```python
from build123d import *

# Parameters (mm, degrees)
SKETCH_1_W          = 86
SKETCH_1_H          = 44.4
EXTRUDE_1_DEPTH     = 19.6
EXTRUDE_2_DEPTH     = 5
SKETCH_3_W          = 83.2
SKETCH_3_H          = 20.402884615
SKETCH_3_H_2        = 20.397115385
CUT_EXTRUDE_1_DEPTH = 18.4
FILLET_1_R          = 3


with BuildPart() as part:
    # Эскиз1 → Бобышка-Вытянуть1 (new body)
    with BuildSketch(Plane.XY):
        Rectangle(SKETCH_1_W, SKETCH_1_H)
    extrude(amount=EXTRUDE_1_DEPTH)

    # Эскиз2 → Бобышка-Вытянуть2 (add)
    with BuildSketch(Plane.XY):
        with BuildLine():
            Line((43, 17.2), (43, 13.108775687))
            ThreePointArc((43, 13.108775687), (53.273546839, 0), (43, -13.108775687))
            Line((43, -13.108775687), (43, -17.2))
            ThreePointArc((43, -17.2), (57.273546839, 0), (43, 17.2))
        make_face()
    extrude(amount=EXTRUDE_2_DEPTH)

    # Эскиз3 → Вырез-Вытянуть1 (cut)
    with BuildSketch(Plane.XY.offset(19.6)):
        with Locations((0.2, 10.798557692)):
            Rectangle(SKETCH_3_W, SKETCH_3_H)
        with Locations((0.2, -10.801442308)):
            Rectangle(SKETCH_3_W, SKETCH_3_H_2)
    extrude(amount=-CUT_EXTRUDE_1_DEPTH, mode=Mode.SUBTRACT)

    # Скругление1
    fillet_1_edges = [part.edges().sort_by_distance(p)[0] for p in [
        (-41.4, 21, 10.4),
        (-41.4, -21, 10.4),
        (-43, -22.2, 9.8),
        (-43, 22.2, 9.8),
    ]]
    fillet(fillet_1_edges, radius=FILLET_1_R)


solid = part.part
```
Read the model definition and answer for the solid it produces. Units are mm, in the model's axes. A direction names the side the tool comes from. Coordinates: 2 decimals unless noted, no trailing zeros. Write each loop counter-clockwise with the first axis right and the second up, starting at its lowest first coordinate (ties: lowest second). Pieces come first, ordered by that corner, then holes. Notation, with made-up numbers: (-17.75, 40) -> (30.25, 40) arc R23 cw to (30.25, 60) -> close; hole circle Ø4 at (8.5, 19). An arc over 180 degrees is marked (long way). Write item = value, one per line.
(1) Section D-D on y = 1.5 is taken. Write down the section's boundary in (x, z).
From the geometry:
outline = (-43, 0) -> (43, 0) -> (43, 19.6) -> (41.8, 19.6) -> (41.8, 1.2) -> (-41.4, 1.2) -> (-41.4, 19.6) -> (-43, 19.6) -> close; (53.19, 0) -> (57.21, 0) -> (57.21, 5) -> (53.19, 5) -> close
(2) For a pull along X with two mould halves and no side action, classify faces 1 (the face through (1, 21, 11)), 2 (the face through (57.27, -0.34, 2.46)), 3 (the face through (-42.14, -21.3, 9.94)), 4 (the face through (1, 22.2, 10)) as +X half, -X half, draft (parallel to the pull), parting line (faces both ways), or undercut.
From the geometry:
face_1 = undercut
face_2 = +X half
face_3 = -X half
face_4 = draft
(3) Straight lines are drawn through the part: L1, parallel to Y at x = 16, z = 10.5; L2, parallel to X at y = 18, z = 12.5; L3, parallel to X at y = 3, z = 2. For each, find the intervals that lie inside material, in ascending order. Write a range as from..to.
From the geometry:
L1 = -22.2..-21, -0.6..0.6, 21..22.2
L2 = -43..-41.4, 41.8..43
L3 = -43..-41.4, 41.8..43, 52.94..57.01
(4) Which of the six approach directions +Z, -Z, +X, -X, +Y, -Y give full straight-line access (tool end or side, diameter ignored) to faces 5 (the face through (-13, 0, 19.6)), 6 (the face through (-40.5, 20.14, 10.27)), 7 (the face through (53.3, -2.5, 5))?
From the geometry:
face_5 = +Z, +X, -X, +Y, -Y
face_6 = +Z
face_7 = +Z, +X, +Y, -Y
(5) Section B-B on z = 8.5 is taken. Write down the section's boundary in (x, y), plus the area to 3 significant figures.
From the geometry:
outline = (-43, -19.2) arc R3 ccw to (-40, -22.2) -> (43, -22.2) -> (43, 22.2) -> (-40, 22.2) arc R3 ccw to (-43, 19.2) -> close; hole (-41.4, -18) arc R3 ccw to (-38.4, -21) -> (41.8, -21) -> (41.8, -0.6) -> (-41.4, -0.6) -> close; hole (-41.4, 0.6) -> (41.8, 0.6) -> (41.8, 21) -> (-38.4, 21) arc R3 ccw to (-41.4, 18) -> close
area = 424 mm2
(6) Section C-C on x = -35.5 is taken. Write down the section's boundary in (y, z).
From the geometry:
outline = (-22.2, 0) -> (22.2, 0) -> (22.2, 19.6) -> (21, 19.6) -> (21, 1.2) -> (0.6, 1.2) -> (0.6, 19.6) -> (-0.6, 19.6) -> (-0.6, 1.2) -> (-21, 1.2) -> (-21, 19.6) -> (-22.2, 19.6) -> close
(7) Section A-A on y = -8 is taken. Write down the section's boundary in (x, z).
From the geometry:
outline = (-43, 0) -> (43, 0) -> (43, 19.6) -> (41.8, 19.6) -> (41.8, 1.2) -> (-41.4, 1.2) -> (-41.4, 19.6) -> (-43, 19.6) -> close; (50.65, 0) -> (55.34, 0) -> (55.34, 5) -> (50.65, 5) -> close
(8) Given pin 1 Ø15.5 at (x, y) = (52.5, -1) entering from +Z; pin 2 Ø6 at (x, y) = (-0.5, 14.5) entering from +Z; pin 3 Ø8.5 at (y, z) = (-6, 10) entering from +X; pin 4 Ø1.5 at (x, y) = (0, 2) entering from -Z, each flat-ended and moving along its own axis, determine where each tip first touches the part or whether it passes through.
From the geometry:
pin_1 = 5
pin_2 = 1.2
pin_3 = 43
pin_4 = 0
